from build123d import *

# Parameters (mm, degrees)
SKETCH006_W     = 31.8
SKETCH006_H     = 19.8
PAD001_DEPTH    = 0.8
SKETCH007_W     = 12
SKETCH007_H     = 4.5
POCKET005_DEPTH = 0.801
SKETCH008_W     = 5
SKETCH008_H     = 1.5
POCKET006_DEPTH = 0.801
FILLET002_R     = 0.5
FILLET003_R     = 0.3


with BuildPart() as part:
    # Sketch006 → Pad001 (new body)
    with BuildSketch(Plane.XY):
        Rectangle(SKETCH006_W, SKETCH006_H)
    extrude(amount=PAD001_DEPTH)

    # Sketch007 (on Face6 of Pad001) → Pocket005 (cut, through all)
    with BuildSketch(Plane.XY.offset(0.8)):
        with Locations((-0.5, 7.65)):
            Rectangle(SKETCH007_W, SKETCH007_H)
    extrude(amount=-POCKET005_DEPTH, mode=Mode.SUBTRACT)

    # Sketch008 (on Face4 of Pocket005) → Pocket006 (cut, through all)
    with BuildSketch(Plane.XY.offset(0.8)):
        with Locations((0, -5.15)):
            Rectangle(SKETCH008_W, SKETCH008_H)
    extrude(amount=-POCKET006_DEPTH, mode=Mode.SUBTRACT)

    # Fillet002
    fillet002_edges = [part.edges().sort_by_distance(p)[0] for p in [
        (15.9, -9.9, 0.4),
        (15.9, 9.9, 0.4),
        (-15.9, 9.9, 0.4),
        (-15.9, -9.9, 0.4),
    ]]
    fillet(fillet002_edges, radius=FILLET002_R)

    # Fillet003
    fillet003_edges = [part.edges().sort_by_distance(p)[0] for p in [
        (-15.9, 0, 0.8),
        (-15.9, 0, 0),
        (-10.95, 9.9, 0),
        (-10.95, 9.9, 0.8),
        (-0.5, 5.4, 0.8),
        (-0.5, 5.4, 0),
        (5.5, 7.65, 0),
        (5.5, 7.65, 0.8),
        (-6.5, 7.65, 0.8),
        (10.45, 9.9, 0),
        (10.45, 9.9, 0.8),
        (15.9, 0, 0.8),
        (15.9, 0, 0),
        (-6.5, 7.65, 0),
    ]]
    fillet(fillet003_edges, radius=FILLET003_R)


solid = part.part
Source: CAD feature listing. Evaluate the final solid. Frame: model axes, mm. Round coordinates to 2 decimals unless told otherwise and drop trailing zeros. Write each loop counter-clockwise with the first axis right and the second up, starting at its lowest first coordinate (ties: lowest second). Pieces come first, ordered by that corner, then holes. Notation, with made-up numbers: (-8.75, 75.25) - (29.25, 75.25) arc R11 cw to (29.25, 94.25) - close; hole circle Ø9 at (-5.5, 22). An arc over 180 degrees is marked (long way). Use CSV: the item, a comma, the result in double quotes. Start each with the question number.
(1) Cut plane B-B, the plane x = -2. Return loops of the section in (y, z), and give its area (3 significant figures).
(2) Cut plane A-A, the plane y = -4.75. Return loops of the section in (x, z), and give its area (3 significant figures).
(3) Cut plane C-C, the plane y = 7.5. Return loops of the section in (x, z), and give its area (3 significant figures).
(4) Material intervals for probe 1 along Y at (x, z) = (-1, 0.3); probe 2 along X at (y, z) = (-5.5, 0.3); probe 3 along X at (y, z) = (7.25, 0.55), sorted ascending. Write a range as [from, to].
Geometry says:
1,outline,"(-9.9, 0.3) arc R0.3 ccw to (-9.6, 0) - (-5.9, 0) - (-5.9, 0.8) - (-9.6, 0.8) arc R0.3 ccw to (-9.9, 0.5) - close; (-4.4, 0) - (5.1, 0) arc R0.3 ccw to (5.4, 0.3) - (5.4, 0.5) arc R0.3 ccw to (5.1, 0.8) - (-4.4, 0.8) - close"
1,area,"11.0 mm²"
2,outline,"(-15.9, 0.3) arc R0.3 ccw to (-15.6, 0) - (-2.5, 0) - (-2.5, 0.8) - (-15.6, 0.8) arc R0.3 ccw to (-15.9, 0.5) - close; (2.5, 0) - (15.6, 0) arc R0.3 ccw to (15.9, 0.3) - (15.9, 0.5) arc R0.3 ccw to (15.6, 0.8) - (2.5, 0.8) - close"
2,area,"21.4 mm²"
3,outline,"(-15.9, 0.3) arc R0.3 ccw to (-15.6, 0) - (-6.8, 0) arc R0.3 ccw to (-6.5, 0.3) - (-6.5, 0.5) arc R0.3 ccw to (-6.8, 0.8) - (-15.6, 0.8) arc R0.3 ccw to (-15.9, 0.5) - close; (5.5, 0.3) arc R0.3 ccw to (5.8, 0) - (15.6, 0) arc R0.3 ccw to (15.9, 0.3) - (15.9, 0.5) arc R0.3 ccw to (15.6, 0.8) - (5.8, 0.8) arc R0.3 ccw to (5.5, 0.5) - close"
3,area,"15.7 mm²"
4,probe 1,"[-9.9, -5.9], [-4.4, 5.4]"
4,probe 2,"[-15.9, -2.5], [2.5, 15.9]"
4,probe 3,"[-15.9, -6.5], [5.5, 15.9]"
